Design review of the part built by this model. Coordinates are the model's own, in mm. A direction names the side the tool comes from. Coordinates: 2 decimals unless noted, no trailing zeros. Loops run counter-clockwise (first coordinate to the right, second up) from the corner with the lowest first, then second, coordinate; pieces in that order, holes last. Notation, with made-up numbers: (40.25, -3.75) -> (44.25, -3.75) arc R8 cw to (44.25, 5.25) -> close; hole circle Ø5 at (53, 12.5). An arc over 180 degrees is marked (long way). Use one line per item in the form item = value. Start each with the question number.
1. Consider section D-D (x = 7). State the section outline as (y, z) points (3 decimals).
2. Consider section B-B (x = -6.5). State the section outline as (y, z) points.
3. The part is to be moulded in two halves that separate along Y. For faces 4 (the face through (15.321, 14.521, 27.793)), 5 (the face through (15, -6, 19.494)), 6 (the face through (14.577, 4.98, 16.913)), 7 (the face through (5.3, 4.325, 20.6)), say which applies: released by +Y, released by -Y, zero draft, split by the parting line, or undercut.
4. Machinability: for faces 1 (the face through (15.32, 11.85, 9.03)), 2 (the face through (15.32, 0.29, 26.84)), 3 (the face through (9, -1, 18)), which of the approach directions +Z, -Z, +X, -X, +Y, -Y give a long, thin tool a straight path to every point of the face, cutting with its end or side? Answer none if there is none.
5. Wall thickness on line 1 (Y direction, x = 15.5, z = 18.25) (3 decimals); line 2 (Y direction, x = 12.5, z = 18.4) (3 decimals); line 3 (Y direction, x = 13.5, z = 18.4) (3 decimals): over which ranges is each line inside the solid? List them lowest first. Write a range as from..to.
6. Consider section C-C (y = -12.5). State the section outline as (x, z) points.
7. Consider section A-A (y = 12). State the section outline as (x, z) points.
8. For pin 1 (10 mm diameter, centred on x = -12.5, z = 11, fed in from -Y); pin 2 (1 mm diameter, centred on y = -4.5, z = 25.5, fed in from +X); pin 3 (0.7 mm diameter, centred on x = 5, z = 20.5, fed in from +Y), all flat-tipped, find the tip position at first contact; note any pin that passes through.
from build123d import *

# Parameters (mm, degrees)
CYLINDER005_R               = 1.5
CYLINDER005_DEPTH           = 30.9
CYLINDER006_R               = 8
CYLINDER006_DEPTH           = 19.6
CUBE008_W                   = 1.7
CUBE008_H                   = 6
CUBE008_DEPTH               = 8
CYLINDER016_R               = 1.25
CYLINDER016_DEPTH           = 1
CYLINDER017_R               = 1.25
CYLINDER017_DEPTH           = 1
CYLINDER017_PLACEMENT_ANGLE = 120
CYLINDER018_R               = 1.25
CYLINDER018_DEPTH           = 1
CYLINDER018_PLACEMENT_ANGLE = 240
CUBE010_W                   = 7
CUBE010_H                   = 2.1875
CUBE010_DEPTH               = 3
CUBE010_PLACEMENT_ANGLE     = 30
CUBE011_W                   = 7
CUBE011_H                   = 2.1875
CUBE011_DEPTH               = 3
CUBE011_PLACEMENT_ANGLE     = 60
CUBE012_W                   = 7
CUBE012_H                   = 2.1875
CUBE012_DEPTH               = 3
CUBE013_W                   = 7
CUBE013_H                   = 2.1875
CUBE013_DEPTH               = 3
CUBE013_PLACEMENT_ANGLE     = 120
CUBE014_W                   = 7
CUBE014_H                   = 2.1875
CUBE014_DEPTH               = 3
CUBE014_PLACEMENT_ANGLE     = 150
CUBE015_W                   = 7
CUBE015_H                   = 2.1875
CUBE015_DEPTH               = 3
CUBE016_W                   = 7
CUBE016_H                   = 2.1875
CUBE016_DEPTH               = 3
CUBE016_PLACEMENT_ANGLE     = 210
CUBE017_W                   = 7
CUBE017_H                   = 2.1875
CUBE017_DEPTH               = 3
CUBE017_PLACEMENT_ANGLE     = 240
CUBE018_W                   = 7
CUBE018_H                   = 2.1875
CUBE018_DEPTH               = 3
CUBE019_W                   = 7
CUBE019_H                   = 2.1875
CUBE019_DEPTH               = 3
CUBE019_PLACEMENT_ANGLE     = 60
CUBE020_W                   = 7
CUBE020_H                   = 2.1875
CUBE020_DEPTH               = 3
CUBE020_PLACEMENT_ANGLE     = 30
CUBE021_W                   = 7
CUBE021_H                   = 2.1875
CUBE021_DEPTH               = 3
CUBE009_W                   = 7
CUBE009_H                   = 2.1875
CUBE009_DEPTH               = 3
CYLINDER015_R               = 1.7
CYLINDER015_DEPTH           = 22.4
CYLINDER009_R               = 3
CYLINDER009_DEPTH           = 0.5
CYLINDER010_R               = 2.8
CYLINDER010_DEPTH           = 11.2
CYLINDER011_R               = 4
CYLINDER011_DEPTH           = 7
CYLINDER013_R               = 4
CYLINDER013_DEPTH           = 8
CYLINDER012_R               = 4.8
CYLINDER012_DEPTH           = 8
CYLINDER014_R               = 13.25
CYLINDER014_DEPTH           = 3
CYLINDER019_R               = 1.5
CYLINDER019_DEPTH           = 19
CYLINDER007_R               = 7.7
CYLINDER007_DEPTH           = 3
CYLINDER004_R               = 6.75
CYLINDER004_DEPTH           = 4
GROUP004_ROLL_ANGLE         = -90
GROUP004_PLACEMENT_ANGLE    = 90


with BuildPart() as cylinder005:
    # cylinder005 → cylinder005 (new body)
    with BuildSketch(Plane.XY.offset(-3.8)):
        Circle(CYLINDER005_R)
    extrude(amount=CYLINDER005_DEPTH)


with BuildPart() as cylinder006:
    # cylinder006 → cylinder006 (new body)
    with BuildSketch(Plane.XY.offset(4)):
        Circle(CYLINDER006_R)
    extrude(amount=CYLINDER006_DEPTH)


with BuildPart() as cube008:
    # cube008 → cube008 (new body)
    with BuildSketch(Plane(origin=(-0.85, -3, 8), x_dir=(1, 0, 0), z_dir=(0, 0, 1))):
        with Locations((0.85, 3)):
            Rectangle(CUBE008_W, CUBE008_H)
    extrude(amount=CUBE008_DEPTH)


with BuildPart() as cylinder016:
    # cylinder016 → cylinder016 (new body)
    with BuildSketch(Plane(origin=(4.4, 0, 7), x_dir=(1, 0, 0), z_dir=(0, 0, 1))):
        Circle(CYLINDER016_R)
    extrude(amount=CYLINDER016_DEPTH)


with BuildPart() as cylinder017:
    # cylinder017 → cylinder017 (new body)
    with BuildSketch(Plane.XY):
        Circle(CYLINDER017_R)
    extrude(amount=CYLINDER017_DEPTH)


with BuildPart() as cylinder017_1:
    # cylinder017 placement: moved
    add(cylinder017.part.moved(Location((-2.2, 3.810512, 7))).rotate(Axis((-2.2, 3.810512, 7), (0, 0, 1)), CYLINDER017_PLACEMENT_ANGLE))


with BuildPart() as cylinder018:
    # cylinder018 → cylinder018 (new body)
    with BuildSketch(Plane.XY):
        Circle(CYLINDER018_R)
    extrude(amount=CYLINDER018_DEPTH)


with BuildPart() as cylinder018_1:
    # cylinder018 placement: moved
    add(cylinder018.part.moved(Location((-2.2, -3.810512, 7))).rotate(Axis((-2.2, -3.810512, 7), (0, 0, 1)), CYLINDER018_PLACEMENT_ANGLE))


with BuildPart() as cube010:
    # cube010 → cube010 (new body)
    with BuildSketch(Plane.XY):
        with Locations((3.5, 1.09375)):
            Rectangle(CUBE010_W, CUBE010_H)
    extrude(amount=CUBE010_DEPTH)


with BuildPart() as cube010_1:
    # cube010 placement: moved
    add(cube010.part.moved(Location((8.990623, 3.927785, 0))).rotate(Axis((8.990623, 3.927785, 0), (0, 0, 1)), CUBE010_PLACEMENT_ANGLE))


with BuildPart() as cube011:
    # cube011 → cube011 (new body)
    with BuildSketch(Plane.XY):
        with Locations((3.5, 1.09375)):
            Rectangle(CUBE011_W, CUBE011_H)
    extrude(amount=CUBE011_DEPTH)


with BuildPart() as cube011_1:
    # cube011 placement: moved
    add(cube011.part.moved(Location((5.822215, 7.896873, 0))).rotate(Axis((5.822215, 7.896873, 0), (0, 0, 1)), CUBE011_PLACEMENT_ANGLE))


with BuildPart() as cube012:
    # cube012 → cube012 (new body)
    with BuildSketch(Plane(origin=(1.09375, 9.75, 0), x_dir=(0, 1, 0), z_dir=(0, 0, 1))):
        with Locations((3.5, 1.09375)):
            Rectangle(CUBE012_W, CUBE012_H)
    extrude(amount=CUBE012_DEPTH)


with BuildPart() as cube013:
    # cube013 → cube013 (new body)
    with BuildSketch(Plane.XY):
        with Locations((3.5, 1.09375)):
            Rectangle(CUBE013_W, CUBE013_H)
    extrude(amount=CUBE013_DEPTH)


with BuildPart() as cube013_1:
    # cube013 placement: moved
    add(cube013.part.moved(Location((-3.927785, 8.990623, 0))).rotate(Axis((-3.927785, 8.990623, 0), (0, 0, 1)), CUBE013_PLACEMENT_ANGLE))


with BuildPart() as cube014:
    # cube014 → cube014 (new body)
    with BuildSketch(Plane.XY):
        with Locations((3.5, 1.09375)):
            Rectangle(CUBE014_W, CUBE014_H)
    extrude(amount=CUBE014_DEPTH)


with BuildPart() as cube014_1:
    # cube014 placement: moved
    add(cube014.part.moved(Location((-7.896873, 5.822215, 0))).rotate(Axis((-7.896873, 5.822215, 0), (0, 0, 1)), CUBE014_PLACEMENT_ANGLE))


with BuildPart() as cube015:
    # cube015 → cube015 (new body)
    with BuildSketch(Plane(origin=(-9.75, 1.09375, 0), x_dir=(-1, 0, 0), z_dir=(0, 0, 1))):
        with Locations((3.5, 1.09375)):
            Rectangle(CUBE015_W, CUBE015_H)
    extrude(amount=CUBE015_DEPTH)


with BuildPart() as cube016:
    # cube016 → cube016 (new body)
    with BuildSketch(Plane.XY):
        with Locations((3.5, 1.09375)):
            Rectangle(CUBE016_W, CUBE016_H)
    extrude(amount=CUBE016_DEPTH)


with BuildPart() as cube016_1:
    # cube016 placement: moved
    add(cube016.part.moved(Location((-8.990623, -3.927785, 0))).rotate(Axis((-8.990623, -3.927785, 0), (0, 0, 1)), CUBE016_PLACEMENT_ANGLE))


with BuildPart() as cube017:
    # cube017 → cube017 (new body)
    with BuildSketch(Plane.XY):
        with Locations((3.5, 1.09375)):
            Rectangle(CUBE017_W, CUBE017_H)
    extrude(amount=CUBE017_DEPTH)


with BuildPart() as cube017_1:
    # cube017 placement: moved
    add(cube017.part.moved(Location((-5.822215, -7.896873, 0))).rotate(Axis((-5.822215, -7.896873, 0), (0, 0, 1)), CUBE017_PLACEMENT_ANGLE))


with BuildPart() as cube018:
    # cube018 → cube018 (new body)
    with BuildSketch(Plane(origin=(-1.09375, -9.75, 0), x_dir=(0, -1, 0), z_dir=(0, 0, 1))):
        with Locations((3.5, 1.09375)):
            Rectangle(CUBE018_W, CUBE018_H)
    extrude(amount=CUBE018_DEPTH)


with BuildPart() as cube019:
    # cube019 → cube019 (new body)
    with BuildSketch(Plane.XY):
        with Locations((3.5, 1.09375)):
            Rectangle(CUBE019_W, CUBE019_H)
    extrude(amount=CUBE019_DEPTH)


with BuildPart() as cube019_1:
    # cube019 placement: moved
    add(cube019.part.moved(Location((3.927785, -8.990623, 0))).rotate(Axis((3.927785, -8.990623, 0), (0, 0, -1)), CUBE019_PLACEMENT_ANGLE))


with BuildPart() as cube020:
    # cube020 → cube020 (new body)
    with BuildSketch(Plane.XY):
        with Locations((3.5, 1.09375)):
            Rectangle(CUBE020_W, CUBE020_H)
    extrude(amount=CUBE020_DEPTH)


with BuildPart() as cube020_1:
    # cube020 placement: moved
    add(cube020.part.moved(Location((7.896873, -5.822215, 0))).rotate(Axis((7.896873, -5.822215, 0), (0, 0, -1)), CUBE020_PLACEMENT_ANGLE))


with BuildPart() as cube021:
    # cube021 → cube021 (new body)
    with BuildSketch(Plane(origin=(9.75, -1.09375, 0), x_dir=(1, 0, 0), z_dir=(0, 0, 1))):
        with Locations((3.5, 1.09375)):
            Rectangle(CUBE021_W, CUBE021_H)
    extrude(amount=CUBE021_DEPTH)


with BuildPart() as group003:
    # cube009 → cube009 (new body)
    with BuildSketch(Plane(origin=(9.75, -1.09375, 0), x_dir=(1, 0, 0), z_dir=(0, 0, 1))):
        with Locations((3.5, 1.09375)):
            Rectangle(CUBE009_W, CUBE009_H)
    extrude(amount=CUBE009_DEPTH)

    # Group003: union cube010, cube011, cube012, cube013, cube014, cube015, cube016, cube017, cube018, cube019, cube020, cube021
    add(cube010_1.part)
    add(cube011_1.part)
    add(cube012.part)
    add(cube013_1.part)
    add(cube014_1.part)
    add(cube015.part)
    add(cube016_1.part)
    add(cube017_1.part)
    add(cube018.part)
    add(cube019_1.part)
    add(cube020_1.part)
    add(cube021.part)


with BuildPart() as union002:
    # cylinder015 → cylinder015 (new body)
    with BuildSketch(Plane.XY):
        Circle(CYLINDER015_R)
    extrude(amount=CYLINDER015_DEPTH)

    # union002: union cube008, cylinder016, cylinder017, cylinder018, Group003
    add(cube008.part)
    add(cylinder016.part)
    add(cylinder017_1.part)
    add(cylinder018_1.part)
    add(group003.part)


with BuildPart() as cylinder009:
    # cylinder009 → cylinder009 (new body)
    with BuildSketch(Plane.XY.offset(11.2)):
        Circle(CYLINDER009_R)
    extrude(amount=CYLINDER009_DEPTH)


with BuildPart() as cylinder010:
    # cylinder010 → cylinder010 (new body)
    with BuildSketch(Plane.XY):
        Circle(CYLINDER010_R)
    extrude(amount=CYLINDER010_DEPTH)


with BuildPart() as cylinder011:
    # cylinder011 → cylinder011 (new body)
    with BuildSketch(Plane.XY):
        Circle(CYLINDER011_R)
    extrude(amount=CYLINDER011_DEPTH)


with BuildPart() as cylinder013:
    # cylinder013 → cylinder013 (new body)
    with BuildSketch(Plane.XY):
        Circle(CYLINDER013_R)
    extrude(amount=CYLINDER013_DEPTH)


with BuildPart() as difference001:
    # cylinder012 → cylinder012 (new body)
    with BuildSketch(Plane.XY):
        Circle(CYLINDER012_R)
    extrude(amount=CYLINDER012_DEPTH)

    # difference001: cut cylinder013
    add(cylinder013.part, mode=Mode.SUBTRACT)


with BuildPart() as cylinder014:
    # cylinder014 → cylinder014 (new body)
    with BuildSketch(Plane.XY):
        Circle(CYLINDER014_R)
    extrude(amount=CYLINDER014_DEPTH)


with BuildPart() as difference002:
    # cylinder008 → cylinder008 (revolve)
    with BuildSketch(Plane(origin=(0, 0, 11.7), x_dir=(1, 0, 0), z_dir=(0, -1, 0))):
        Polygon((0, 0), (3, 0), (2.6, 0.5), (0, 0.5), align=None)
    revolve(axis=Axis((0, 0, 11.7), (0, 0, 1)))

    # union001: union cylinder009, cylinder010, cylinder011, difference001, cylinder014
    add(cylinder009.part)
    add(cylinder010.part)
    add(cylinder011.part)
    add(difference001.part)
    add(cylinder014.part)

    # difference002: cut union002
    add(union002.part, mode=Mode.SUBTRACT)


with BuildPart() as difference002_1:
    # difference002 placement: moved
    add(difference002.part.moved(Location((0, 0, -7.8))))


with BuildPart() as cylinder019:
    # cylinder019 → cylinder019 (new body)
    with BuildSketch(Plane.XY.offset(-11)):
        Circle(CYLINDER019_R)
    extrude(amount=CYLINDER019_DEPTH)


with BuildPart() as matrix_union:
    # cylinder007 → cylinder007 (new body)
    with BuildSketch(Plane.XY):
        Circle(CYLINDER007_R)
    extrude(amount=CYLINDER007_DEPTH)

    # Matrix_Union: union difference002, cylinder019
    add(difference002_1.part)
    add(cylinder019.part)


with BuildPart() as matrix_union_1:
    # Matrix_Union placement: moved
    add(matrix_union.part.moved(Location((13.175, 0, 0))))


with BuildPart() as obj1:
    # cylinder004 → cylinder004 (new body)
    with BuildSketch(Plane.XY):
        Circle(CYLINDER004_R)
    extrude(amount=CYLINDER004_DEPTH)

    # Group004: union cylinder005, cylinder006, Matrix_Union
    add(cylinder005.part)
    add(cylinder006.part)
    add(matrix_union_1.part)


with BuildPart() as obj1_1:
    # Group004 roll: moved
    add(obj1.part.rotate(Axis((0, 0, 0), (1, 0, 0)), GROUP004_ROLL_ANGLE))


with BuildPart() as obj1_2:
    # Group004 placement: moved
    add(obj1_1.part.moved(Location((9, -8, 18.4))).rotate(Axis((9, -8, 18.4), (0, 0, 1)), GROUP004_PLACEMENT_ANGLE))


solid = obj1_2.part
Geometry check:
q1.outline = (-1.933, 15.44) arc R7.7 ccw (long way) to (-1.933, 21.36) arc R6.75 ccw (long way) to start
q2.outline = circle Ø16 at (-8, 18.4)
q3.face_4 = released by +Y
q3.face_5 = zero draft
q3.face_6 = undercut
q3.face_7 = undercut
q4.face_1 = -Z, +X, -X
q4.face_2 = +X, -X
q4.face_3 = none
q5.line_1 = -4.575..3.482, 3.683..6.667, 6.868..14.925
q5.line_2 = -9.5..-6.5, 0.375..3.475, 3.675..6.675, 6.875..9.975
q5.line_3 = 0.375..3.475, 3.675..6.675, 6.875..9.975
q6.outline = (-14.6, 11.79) -> (5, 11.79) -> (5, 13.37) -> (9, 13.37) -> (9, 23.43) -> (5, 23.43) -> (5, 25.01) -> (-14.6, 25.01) -> close
q7.outline = (6, 14.83) -> (9, 14.83) -> (9, 21.97) -> (6, 21.97) -> close; (13.8, 8.77) -> (16.8, 8.77) -> (16.8, 28.03) -> (13.8, 28.03) -> close
q8.pin_1 = -15.63
q8.pin_2 = 16.8
q8.pin_3 = 7.6
